Autodesk Inventor part; units mm, degrees
ref_plane "YZ Plane" through (0, 0, 0) normal (1, 0, 0) x (0, 1, 0)
ref_plane "XZ Plane" through (0, 0, 0) normal (0, 1, 0) x (-1, 0, 0)
ref_plane "XY Plane" through (0, 0, 0) normal (0, 0, 1) x (1, 0, 0)
sketch "Sketch1" plane through (0, 0, 0) normal (0, 0, 1) x (1, 0, 0)
  circle A0 centre (0, 0) radius 0.635
  line L0 (-1.905, 2.54) -> (-5.08, 27.94)
  line L1 (5.08, 27.94) -> (1.905, 2.54)
  line L2 (-5.08, -27.94) -> (-1.905, -2.54)
  line L3 (1.905, -2.54) -> (5.08, -27.94)
  arc A1 (-5.08, -27.94) -> (5.08, -27.94) centre (0, -28.575) ccw
  arc A2 (5.08, 27.94) -> (-5.08, 27.94) centre (0, 28.575) ccw
  arc A3 (-1.905, 2.54) -> (-1.905, -2.54) centre (0, 0) ccw
  arc A4 (1.905, -2.54) -> (1.905, 2.54) centre (0, 0) ccw
  dimension "d0" = 1.27
  dimension "d3" = 2.54
  dimension "d4" = 1.905
  dimension "d5" = 2.54
  dimension "d6" = 1.905
  dimension "d7" = 25.4
  dimension "d8" = 25.4
  dimension "d9" = 3.175
  dimension "d10" = 3.175
  dimension "d11" = 25.4
  dimension "d12" = 25.4
  dimension "d13" = 3.175
  dimension "d14" = 3.175
extrude "Extrusion1" add sketch "Sketch1" along normal blind 3.175
fillet "Fillet1" radius 1.27 16 edges at (0, 33.6945, 3.175) (-3.4925, 15.24, 3.175) (3.4925, 15.24, 3.175) (0, -33.6945, 3.175) (-3.4925, -15.24, 3.175) (3.4925, -15.24, 3.175) (0, -33.6945, 0) (-3.4925, -15.24, 0) (3.4925, -15.24, 0) (0, 33.6945, 0) (-3.4925, 15.24, 0) (3.4925, 15.24, 0) (3.175, 0, 3.175) (-3.175, 0, 3.175) (3.175, 0, 0) (-3.175, 0, 0)
properties part number "Prop" material "Nylon 6/6"
Could you check a few things on this model? Use its own coordinates, in mm. A direction names the side the tool comes from. Coordinates: 2 decimals unless noted, no trailing zeros.
Q1. Please list where these lines run through material, in increasing order: L1, parallel to Z at x = -4, y = 31.5; L2, parallel to Z at x = 1.75, y = 10.5; L3, parallel to Y at x = -0.25, z = 1.3.
Q2. Thinking about a two-plate mould opening in X: for faces 1 (the cylindrical face through (-0.08, -0.63, 1.57)), 2 (the cylindrical face through (3.1, 15.03, 0.38)), 3 (the cylindrical face through (-3.056, 14.666, 0.382)), which applies, released by +X, released by -X, zero draft, split by the parting line, or undercut?
Q3. Will this pin go through, and if not, where does the flat tip stop? pin 1 (5 mm diameter, centred on x = -3.5, y = 22, fed in from +Z) (3 decimals).
Q4. Which directions (+Z, -Z, +X, -X, +Y, -Y) give clear straight access to the entire face, cutting with the end or side of a thin tool? Please do faces 4 (the cylindrical face through (3.056, -14.666, 0.382)), 5 (the flat face through (-3.515, -15.418, 1.583)), 6 (the cylindrical face through (-3.04, 14.67, 2.81)), 7 (the cylindrical face through (3.082, 15.036, 2.813)), 8 (the flat face through (3.47, -15.06, 1.58)).
Q5. Suppose I cut it at A-A on x = -2.5. Give the number of separate pieces and of enclosed holes in the cut face, and give its area (3 significant figures).
Answer:
1. L1: z = 0.65 to 2.53
1. L2: z = 0.01 to 3.17
1. L3: y = -33.69 to -0.58, 0.58 to 33.69
2. face 1: undercut
2. face 2: released by +X
2. face 3: released by -X
3. pin 1: stops at z = 3.175
4. face 4: -Z, +X
4. face 5: +Z, -Z, -X
4. face 6: +Z, -X
4. face 7: +Z, +X
4. face 8: +Z, -Z, +X
5. separate pieces: 3
5. enclosed holes: 0
5. area: 160 mm2
